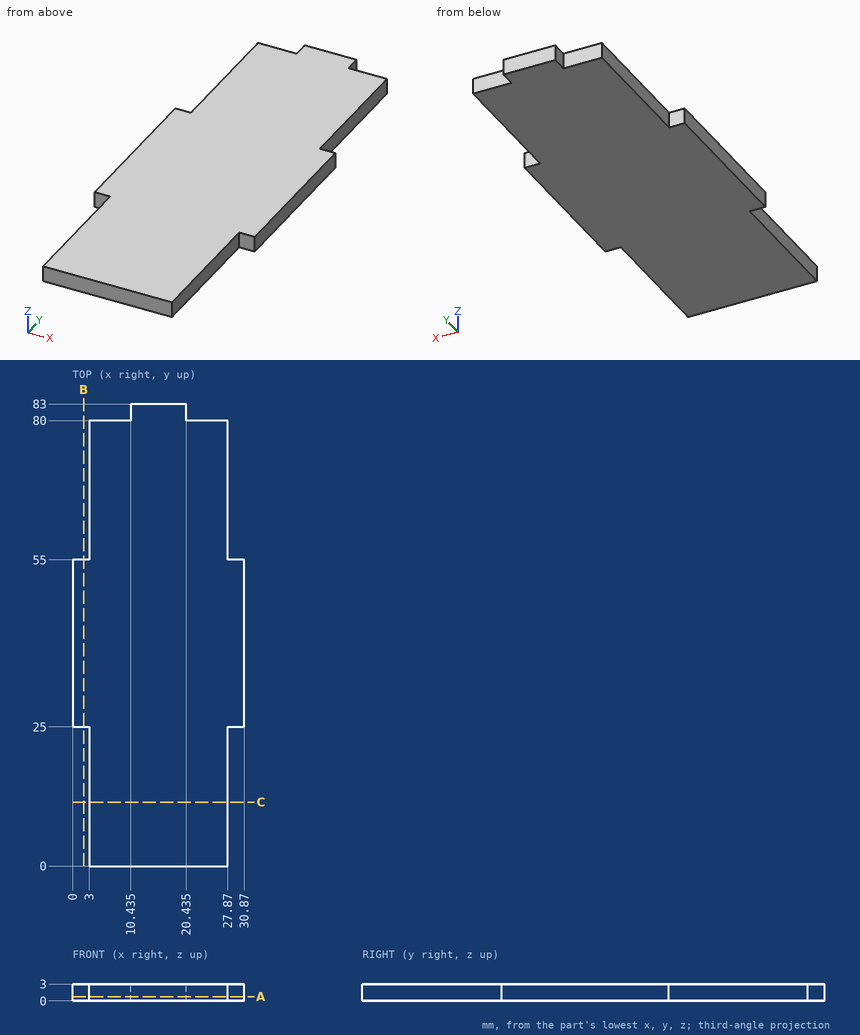
Source: three-view drawing plus pictorial views. Frame: mm from the lowest corner of the part. Round coordinates to 2 decimals unless told otherwise and drop trailing zeros. Order: outer loops, then holes, each group sorted by start corner. A loop starts at its lowest first (then second) coordinate and runs counter-clockwise, first axis right, second up. Notation, with made-up numbers: (38, 37) -> (62, 37) arc R21 ccw to (62, 41) -> close; hole circle Ø8 at (64.25, -17.75). An arc over 180 degrees is marked (long way). Use CSV: the item, a comma, the result in double quotes. Start each with the question number.
1) Material intervals for line 1 along Y through (x, z) = (4, 0.3); line 2 along X through (y, z) = (8, 1.35), sorted ascending. Write a range as from..to.
2) Section C-C (y = 11.5). Return the cut outline in (x, z), and give its area (3 significant figures).
3) First-contact query: pin 1 Ø1.5 at (x, z) = (8, 1.5) entering from +Y; pin 2 Ø1 at (x, z) = (13, 1.5) entering from -Y; pin 3 Ø0.9 at (y, z) = (82, 1.5) entering from -X (3 decimals); pin 4 Ø0.9 at (x, z) = (1.5, 1) entering from -Y. Flat tips, straight axial feed; report the tip coordinate or a pass-through.
4) Section B-B (x = 2). Return the cut outline in (y, z).
5) Section A-A (z = 0.75). Return the cut outline in (x, y) (3 decimals).
Returned:
1,line 1,"y = 0..80"
1,line 2,"x = 3..27.87"
2,outline,"(3, 0) -> (27.87, 0) -> (27.87, 3) -> (3, 3) -> close"
2,area,"74.6 mm²"
3,pin 1,"stops at y = 80"
3,pin 2,"stops at y = 0"
3,pin 3,"stops at x = 10.435"
3,pin 4,"stops at y = 25"
4,outline,"(25, 0) -> (55, 0) -> (55, 3) -> (25, 3) -> close"
5,outline,"(0, 25) -> (3, 25) -> (3, 0) -> (27.87, 0) -> (27.87, 25) -> (30.87, 25) -> (30.87, 55) -> (27.87, 55) -> (27.87, 80) -> (20.435, 80) -> (20.435, 83) -> (10.435, 83) -> (10.435, 80) -> (3, 80) -> (3, 55) -> (0, 55) -> close"
